from build123d import *

# Parameters (mm, degrees)
F1_DEPTH = 43.815
F4_DEPTH = 36.0426
F7_DEPTH = 36.0426


with BuildPart() as f1:
    # F0 (on Top) → F1 (new body, symmetric)
    with BuildSketch(Plane.XY):
        Polygon((1.111168, 37.515668), (-59.248378, 79.779877), (-90.998378, 79.779877), (-90.998378, 26.008077), (-72.787326, 0), (-71.009326, 0), (-71.009326, -2.286), (-72.279326, -2.286), (-90.490378, -28.294077), (-90.490378, -82.116677), (-44.516378, -82.116677), (1.778, -49.701005), (1.778, -47.923005), (4.064, -47.923005), (4.064, -49.193005), (50.358378, -81.608677), (96.332378, -81.608677), (96.332378, -37.895277), (73.022231, -4.604938), (71.244231, -4.604938), (71.244231, -2.318938), (72.514231, -2.318938), (95.824378, 30.971401), (95.824378, 79.739401), (64.109252, 79.779877), (3.397168, 38.023668), (3.397168, 36.245668), (1.111168, 36.245668), align=None)
    extrude(amount=F1_DEPTH, both=True)

    # F3 (on offset) → F4 (cut)
    with BuildSketch(Plane.XY.offset(44.196)):
        Polygon((81.455968, 65.370991), (64.109252, 65.301877), (1.111168, 21.767668), (-59.248378, 65.301877), (-76.629968, 65.411468), (-76.520378, 26.008077), (-56.531326, -2.286), (-76.012378, -28.294077), (-76.121968, -67.748268), (-44.516378, -67.638677), (4.064, -34.715005), (50.358378, -67.130677), (81.963968, -67.240268), (81.854378, -37.895277), (56.766231, -4.604938), (81.346378, 30.971401), align=None)
    extrude(amount=-F4_DEPTH, mode=Mode.SUBTRACT)

    # F6 (on offset) → F7 (cut)
    with BuildSketch(Plane.XY.offset(-44.196)):
        Polygon((-76.012378, -28.294077), (-76.121968, -67.748268), (-44.516378, -67.638677), (4.064, -33.445005), (50.358378, -67.130677), (81.963968, -67.240268), (81.854378, -37.895277), (56.766231, -4.604938), (81.346378, 30.971401), (81.455968, 65.370991), (64.109252, 65.301877), (1.111168, 21.767668), (-59.248378, 65.301877), (-76.629968, 65.411468), (-76.520378, 26.008077), (-56.531326, 0), align=None)
    extrude(amount=F7_DEPTH, mode=Mode.SUBTRACT)


solid = f1.part
CAD build for the part. Positions are in the model's coordinates, mm. A direction names the side the tool comes from. Coordinates: 2 decimals unless noted, no trailing zeros. Order: outer loops, then holes, each group sorted by start corner. A loop starts at its lowest first (then second) coordinate and runs counter-clockwise, first axis right, second up. Notation, with made-up numbers: (-27.75, 47) -> (12.25, 47) arc R7 ccw to (12.25, 60) -> close; hole circle Ø4 at (-18, -0.75). An arc over 180 degrees is marked (long way). Answer in a Markdown table with one row per item.
1) Flat gauge pins, fed straight in: P1, Ø0.6, axis at x = 71.5, z = 13, coming from the -Y side; P2, Ø12, axis at x = -1.5, z = -15, coming from the +Y side; P3, Ø1.1, axis at x = 2, z = -11, coming from the +Y side. Where does each tip first touch, or does it go through?
Check values:
| item | result |
|---|---|
| P1 | y = -81.61 |
| P2 | y = 43.55 |
| P3 | y = 36.25 |
2) Drill centre lines: line 1 (Y direction, x = -73.5, z = -31); line 2 (Y direction, x = 70.5, z = 14.5); line 3 (Y direction, x = -60, z = 28). Where is each one in solid material? Low to high.
Check values:
| item | result |
|---|---|
| line 1 | -82.12 to -67.74, -24.65 to -4.03, 1.02 to 22.08, 65.39 to 79.78 |
| line 2 | -81.61 to -67.2, -22.83 to 15.27, 65.33 to 79.77 |
| line 3 | -82.12 to -67.69, -6.92 to 2.62, 65.31 to 79.78 |
3) Band-saw the part on A-A (x = 77). List the corners of the cut face in (y, z) (3 decimals).
Check values:
| item | result |
|---|---|
| outline | (-81.609, -43.815) -> (-67.223, -43.815) -> (-67.223, -8.153) -> (-31.454, -8.153) -> (-31.454, -43.815) -> (-10.286, -43.815) -> (-10.286, 43.815) -> (-31.454, 43.815) -> (-31.454, 8.153) -> (-67.223, 8.153) -> (-67.223, 43.815) -> (-81.609, 43.815) -> close; (4.087, -43.815) -> (24.681, -43.815) -> (24.681, -8.153) -> (65.353, -8.153) -> (65.353, -43.815) -> (79.763, -43.815) -> (79.763, 43.815) -> (65.353, 43.815) -> (65.353, 8.153) -> (24.681, 8.153) -> (24.681, 43.815) -> (4.087, 43.815) -> close |
4) Band-saw the part on B-B (y = -56). List the corners of the cut face in (x, z) (3 decimals), and give its area (3 significant figures).
Check values:
| item | result |
|---|---|
| outline | (-90.49, -43.815) -> (-76.089, -43.815) -> (-76.089, -8.153) -> (-27.981, -8.153) -> (-27.981, -43.815) -> (-7.218, -43.815) -> (-7.218, 43.815) -> (-27.343, 43.815) -> (-27.343, 8.153) -> (-76.089, 8.153) -> (-76.089, 43.815) -> (-90.49, 43.815) -> close; (13.785, -43.815) -> (35.061, -43.815) -> (35.061, -8.153) -> (81.922, -8.153) -> (81.922, -43.815) -> (96.332, -43.815) -> (96.332, 43.815) -> (81.922, 43.815) -> (81.922, 8.153) -> (34.462, 8.153) -> (34.462, 43.815) -> (13.785, 43.815) -> close |
| area | 7,710 mm2 |
5) Band-saw the part on D-D (y = 12.5). List the corners of the cut face in (x, z) (3 decimals).
Check values:
| item | result |
|---|---|
| outline | (-81.54, -43.815) -> (-66.138, -43.815) -> (-66.138, -8.153) -> (68.584, -8.153) -> (68.584, -43.815) -> (82.891, -43.815) -> (82.891, 43.815) -> (68.584, 43.815) -> (68.584, 8.153) -> (-66.977, 8.153) -> (-66.977, 43.815) -> (-81.54, 43.815) -> close |
6) Band-saw the part on C-C (x = 43). List the corners of the cut face in (y, z) (3 decimals).
Check values:
| item | result |
|---|---|
| outline | (-76.456, -43.815) -> (-61.776, -43.815) -> (-61.776, -8.153) -> (50.715, -8.153) -> (50.715, -43.815) -> (65.261, -43.815) -> (65.261, 43.815) -> (50.715, 43.815) -> (50.715, 8.153) -> (-61.978, 8.153) -> (-61.978, 43.815) -> (-76.456, 43.815) -> close |
7) Which spindle directions (+Z, -Z, +X, -X, +Y, -Y) get a long thin tool onto all of the face, cutting with end or side? Do faces 1 (the face through (26.887, -50.052, -26.234)), 2 (the face through (-21.693, -66.136, 0.613)), 3 (the face through (2, 0, 8.153)). Say none if no direction does.
Check values:
| item | result |
|---|---|
| face 1 | -Z |
| face 2 | +Z, -Z, -Y |
| face 3 | +Z |
